from build123d import *

# Parameters (mm, degrees)
SKETCH1_R           = 1.5
SKETCH1_R_2         = 1
BOSS_EXTRUDE1_DEPTH = 3
FILLET1_R           = 5


with BuildPart() as part:
    # Sketch1 → Boss-Extrude1 (new body)
    with BuildSketch(Plane.XY):
        Polygon((85, 30), (85, 20), (88, 20), (88, 10), (85, 10), (85, 0), (0, 0), (0, 30), align=None)
        with Locations((15, 15)):
            Circle(SKETCH1_R, mode=Mode.SUBTRACT)
        with Locations((7.5, 15)):
            Circle(SKETCH1_R_2, mode=Mode.SUBTRACT)
        with Locations((9.696699141, 20.303300859)):
            Circle(SKETCH1_R_2, mode=Mode.SUBTRACT)
        with Locations((15, 22.5)):
            Circle(SKETCH1_R_2, mode=Mode.SUBTRACT)
        with Locations((20.303300859, 20.303300859)):
            Circle(SKETCH1_R_2, mode=Mode.SUBTRACT)
        with Locations((22.5, 15)):
            Circle(SKETCH1_R_2, mode=Mode.SUBTRACT)
        with Locations((20.303300859, 9.696699141)):
            Circle(SKETCH1_R_2, mode=Mode.SUBTRACT)
        with Locations((15, 7.5)):
            Circle(SKETCH1_R_2, mode=Mode.SUBTRACT)
        with Locations((9.696699141, 9.696699141)):
            Circle(SKETCH1_R_2, mode=Mode.SUBTRACT)
    extrude(amount=BOSS_EXTRUDE1_DEPTH)

    # Fillet1
    fillet1_edges = [part.edges().sort_by_distance(p)[0] for p in [
        (0, 0, 1.5),
        (0, 30, 1.5),
    ]]
    fillet(fillet1_edges, radius=FILLET1_R)


solid = part.part
Design review of the part built by this model. Coordinates are the model's own, in mm. A direction names the side the tool comes from. Round coordinates to 2 decimals unless told otherwise and drop trailing zeros. Write each loop counter-clockwise with the first axis right and the second up, starting at its lowest first coordinate (ties: lowest second). Pieces come first, ordered by that corner, then holes. Notation, with made-up numbers: (34, 79) - (57, 79) arc R23 cw to (57, 96) - close; hole circle Ø1 at (89, 38.25). An arc over 180 degrees is marked (long way). Use a Markdown table: item, result. Add a question column.
1. We need section B-B (y = 15). State the section outline as (x, z) points.
2. We need section C-C (z = 1.05). Count the separate pieces of the cut face and the enclosed holes in it, then the cut area to 3 significant figures.
3. Clearance check with flat-ended pins moving along their axes: pin 1 (2.5 mm diameter, centred on x = 15, y = 15, fed in from -Z); pin 2 (0.9 mm diameter, centred on y = 24, z = 1, fed in from +X). State where each tip first meets the part, or that it passes through.
4. Wall thickness on probe 1 along Y at (x, z) = (22.5, 0.6); probe 2 along X at (y, z) = (19.75, 2.6); probe 3 along X at (y, z) = (13.75, 1): over which ranges is each line inside the solid? List them lowest first.
5. We need section A-A (x = 22.5). State the section outline as (y, z) points.
6. Mouldability with a two-part tool opening along Y and no side actions: class faces 3 (the face through (1, 2, 2)), 4 (the face through (2, 29, 2)), 5 (the face through (88, 15, 1)), 6 (the face through (7.283, 14.024, 1.479)) as +Y half, -Y half, draft (parallel to the pull), parting line (faces both ways), or undercut.
7. For faces 1 (the face through (45, 15, 3)), 2 (the face through (87, 10, 1)), list the 3-axis set-ups (+Z, -Z, +X, -X, +Y, -Y) from which the entire face can be reached by the end or side of a thin tool; tool diameter is ignored.
8. We need section D-D (y = 28). State the section outline as (x, z) points.
Output:
| question | item | result |
|---|---|---|
| 1 | outline | (0, 0) - (6.5, 0) - (6.5, 3) - (0, 3) - close; (8.5, 0) - (13.5, 0) - (13.5, 3) - (8.5, 3) - close; (16.5, 0) - (21.5, 0) - (21.5, 3) - (16.5, 3) - close; (23.5, 0) - (88, 0) - (88, 3) - (23.5, 3) - close |
| 2 | separate pieces | 1 |
| 2 | enclosed holes | 9 |
| 2 | area | 2,540 mm2 |
| 3 | pin 1 | passes through |
| 3 | pin 2 | stops at x = 85 |
| 4 | probe 1 | y = 0 to 14, 16 to 30 |
| 4 | probe 2 | x = 0 to 8.86, 10.53 to 19.47, 21.14 to 88 |
| 4 | probe 3 | x = 0 to 14.17, 15.83 to 88 |
| 5 | outline | (0, 0) - (14, 0) - (14, 3) - (0, 3) - close; (16, 0) - (30, 0) - (30, 3) - (16, 3) - close |
| 6 | face 3 | -Y half |
| 6 | face 4 | +Y half |
| 6 | face 5 | draft |
| 6 | face 6 | undercut |
| 7 | face 1 | +Z, +X, -X, +Y, -Y |
| 7 | face 2 | +Z, -Z, +X, -Y |
| 8 | outline | (1, 0) - (85, 0) - (85, 3) - (1, 3) - close |
